from build123d import *

# Parameters (mm, degrees)
SKETCH_1_R          = 1.6
EXTRUDE_1_DEPTH     = 12
CUT_EXTRUDE_1_DEPTH = 10


with BuildPart() as part:
    # Эскиз1 → Бобышка-Вытянуть1 (new body)
    with BuildSketch(Plane.XY):
        with BuildLine():
            Line((-57.947933857, 4.999983999), (-27.948022281, 4.999983999))
            Line((-27.948022281, 4.999983999), (-25.768907845, -1.020957985))
            ThreePointArc((-25.768907845, -1.020957985), (-21.600669135, -2.680440009), (-20.445626155, 1.654761283))
            Line((-20.445626155, 1.654761283), (-27.948022281, 12.999984004))
            Line((-27.948022281, 12.999984004), (-57.947933857, 12.999984004))
            Line((-57.947933857, 12.999984004), (-65.450329983, 1.654761282))
            ThreePointArc((-65.450329983, 1.654761282), (-64.295287003, -2.680440008), (-60.127048295, -1.020957985))
            Line((-60.127048295, -1.020957985), (-57.947933857, 4.999983999))
        make_face()
        with Locations((-62.947978069, 0)):
            Circle(SKETCH_1_R, mode=Mode.SUBTRACT)
        with Locations((-22.947978069, 0)):
            Circle(SKETCH_1_R, mode=Mode.SUBTRACT)
    extrude(amount=EXTRUDE_1_DEPTH)

    # Эскиз2 → Вырез-Вытянуть1 (cut)
    with BuildSketch(Plane.XY.offset(12)):
        Polygon((-42.947978069, 12.999984004), (-34.947978069, 12.999984004), (-34.947978069, 10.999984004), (-29.947978069, 10.999984004), (-29.947978069, 6.999984004), (-55.947978069, 6.999984004), (-55.947978069, 10.999984004), (-50.947978069, 10.999984004), (-50.947978069, 12.999984004), align=None)
    extrude(amount=-CUT_EXTRUDE_1_DEPTH, mode=Mode.SUBTRACT)


solid = part.part
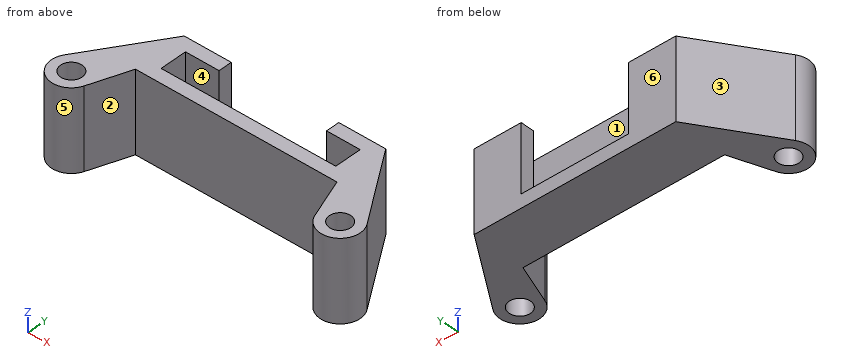
Source: CAD feature listing. Evaluate the final solid. Frame: model axes, mm. Face numbers are marked on the shaded views. A direction names the side the tool comes from. Give positions to 0.01 mm unless a question says otherwise; leave off trailing zeros. Write each loop counter-clockwise with the first axis right and the second up, starting at its lowest first coordinate (ties: lowest second). Pieces come first, ordered by that corner, then holes. Notation, with made-up numbers: M 82.5,70.5 L 119.5,70.5 A21 cw 119.5,100.5 Z; hole C -21,-2 d11. An arc over 180 degrees is marked long. Return JSON: item names as keys, results as strings. Group by question number.
1) Pin query (flat end, axial travel): P1, Ø2.5, axis at x = -54.5, z = 5, coming from the -Y side; P2, Ø1.6, axis at y = 12, z = 4.5, coming from the +X side; P3, Ø5, axis at x = -42, z = 6.5, coming from the +Y side; P4, Ø1.9, axis at x = -22.95, y = 0, coming from the -Z side. Return the tip coordinate at first contact, or that it passes through.
2) Cut plane C-C, the plane y = 3.5. Output: boundary loops of the cut face in (x, z).
3) Cut plane B-B, the plane x = -52. Output: boundary loops of the cut face in (y, z).
4) Cut plane A-A, the plane z = 1.25. Output: boundary loops of the cut face in (x, y).
5) Set-up query: the marked faces 1, 2 and 3. Return all of +Z, -Z, +X, -X, +Y, -Y with unobstructed straight access to the full face (end or side cutting, diameter ignored); none if empty.
6) Cut plane D-D, the plane x = -24. Output: boundary loops of the cut face in (y, z), plus the area to 3 significant figures.
7) Material intervals for line 1 along X through (y, z) = (-1, 10.75); line 2 along Z through (x, y) = (-50, 10); line 3 along Y through (x, z) = (-40, 10), sorted ascending. Write a range as [from, to].
8) Pull-direction query (Y, two-part tool) for the marked faces 4, 5 and 6; classes: pulls with the +Y half, pulls with the -Y half, needs draft (parallel to the pull), parting line crosses it, or undercut.
Recorded:
{
 "1": {"P1": "stops at y = 5", "P2": "stops at x = -26.76", "P3": "stops at y = 7", "P4": "passes through"},
 "2": {"outline": "M -64.23,0 L -58.49,0 L -58.49,12 L -64.23,12 Z; M -27.41,0 L -21.67,0 L -21.67,12 L -27.41,12 Z"},
 "3": {"outline": "M 5,0 L 13,0 L 13,12 L 11,12 L 11,2 L 7,2 L 7,12 L 5,12 Z"},
 "4": {"outline": "M -65.45,1.65 A3 ccw long -60.13,-1.02 L -57.95,5 L -27.95,5 L -25.77,-1.02 A3 ccw long -20.45,1.65 L -27.95,13 L -57.95,13 Z; hole C -62.95,0 d3.2; hole C -22.95,0 d3.2"},
 "5": {"face 1": "+Z", "face 2": "+Z, -Z, -Y", "face 3": "+Z, -Z, -X, +Y"},
 "6": {"outline": "M -2.81,0 L -1.21,0 L -1.21,12 L -2.81,12 Z; M 1.21,0 L 7.03,0 L 7.03,12 L 1.21,12 Z", "area": "89.1 mm²"},
 "7": {"line 1": "x = [-65.78, -64.2], [-61.7, -60.12], [-25.78, -24.2], [-21.7, -20.12]", "line 2": "z = [0, 2]", "line 3": "y = [5, 7]"},
 "8": {"face 4": "undercut", "face 5": "parting line crosses it", "face 6": "pulls with the +Y half"}
}
